Geometry check sheet. Reference: drawing and pictorial views, mm from the part's lowest x, y, z. Give positions to 0.01 mm unless a question says otherwise; leave off trailing zeros. Write each loop counter-clockwise with the first axis right and the second up, starting at its lowest first coordinate (ties: lowest second). Pieces come first, ordered by that corner, then holes.
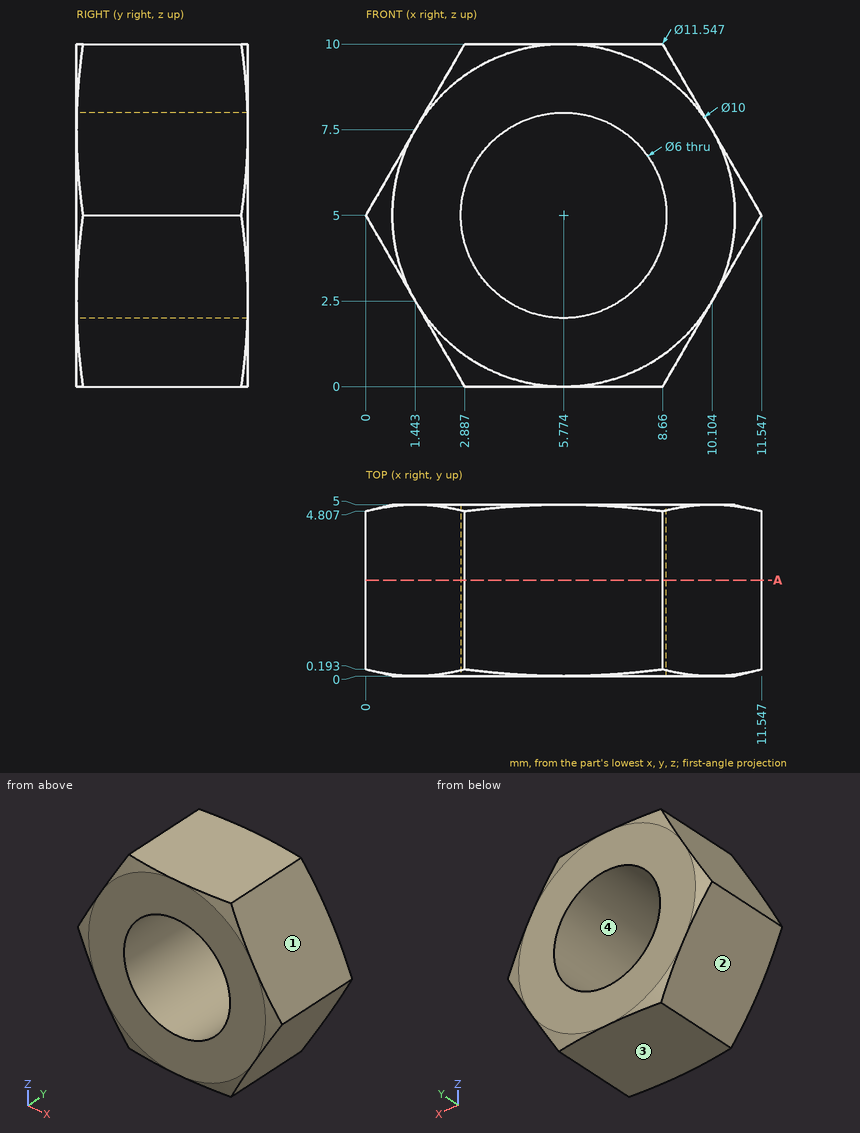
Item 1: Depth check by flat-ended pin: pin 1 (1.5 mm diameter, centred on y = 2, z = 5.5, fed in from +X); pin 2 (1 mm diameter, centred on y = 1.5, z = 7, fed in from +X); pin 3 (2 mm diameter, centred on y = 2, z = 8, fed in from -X) (1 decimal). Enter the tip coordinate at first touch or a pass-through.
Answer key:
pin 1: stops at x = 11.55
pin 2: stops at x = 10.68
pin 3: stops at x = 1.2
Item 2: Sectioned sample at A-A on y = 2.8. Record the cut outline in (x, z).
Answer key:
outline: (0, 5) - (2.89, 0) - (8.66, 0) - (11.55, 5) - (8.66, 10) - (2.89, 10) - close; hole circle Ø6 at (5.77, 5)
Item 3: Scan lines: line 1 along Z through (x, y) = (5.75, 1.2); line 2 along X through (y, z) = (1.1, 3) (1 decimal); line 3 along X through (y, z) = (0.65, 4.75) (1 decimal). Record each from-to range of solid material in increasing order.
Answer key:
line 1: z = 0 to 2, 8 to 10
line 2: x = 1.2 to 3.5, 8 to 10.4
line 3: x = 0.1 to 2.8, 8.8 to 11.4
Item 4: Release check for a two-part mould opening along X. For the marked faces 1, 2, 3 and 4 record: released by +X, released by -X, zero draft, split by the parting line, or undercut.
Answer key:
face 1: released by +X
face 2: released by -X
face 3: zero draft
face 4: undercut
